Could you check a few things on this model? Use its own coordinates, in mm. A direction names the side the tool comes from. Coordinates: 2 decimals unless noted, no trailing zeros. Write each loop counter-clockwise with the first axis right and the second up, starting at its lowest first coordinate (ties: lowest second). Pieces come first, ordered by that corner, then holes.
```python
from build123d import *

# Parameters (mm, degrees)
F2_R     = 1.5
F3_DEPTH = 4
F5_DEPTH = 1.5


with BuildPart() as f1:
    # F0 (on Right) → F1 (revolve)
    with BuildSketch(Plane.YZ):
        with BuildLine():
            Line((0, 0), (0, 6))
            ThreePointArc((0, 6), (-1.1189941578, 3.0922762594), (-1.4995632221, 0))
            Line((-1.4995632221, 0), (0, 0))
        make_face()
    revolve(axis=Axis((0, 0.9339665994, 0), (0, 1, 0)))

    # F2 (on Front) → F3 (join)
    with BuildSketch(Plane.XZ):
        Circle(F2_R)
    extrude(amount=F3_DEPTH)

    # F4 (on Top) → F5 (join, symmetric)
    with BuildSketch(Plane.XY):
        with BuildLine():
            Line((1.4699705266, -3.8650664501), (0, -3.8650664501))
            Line((0, -3.8650664501), (-1.4699705266, -3.8650664501))
            ThreePointArc((-1.4699705266, -3.8650664501), (-2.105403361, -4.0929103047), (-2.4512772628, -4.6726162242))
            Line((-2.4512772628, -4.6726162242), (-5.0702010152, -18.0265497334))
            ThreePointArc((-5.0702010152, -18.0265497334), (-5.0479765813, -18.5021273815), (-4.8083588564, -18.913529096))
            Line((-4.8083588564, -18.913529096), (-2.5877873591, -21.213825008))
            ThreePointArc((-2.5877873591, -21.213825008), (-2.2591365885, -21.4397656254), (-1.8683227817, -21.5192958713))
            Line((-1.8683227817, -21.5192958713), (0, -21.5192958713))
            Line((0, -21.5192958713), (1.8683227817, -21.5192958713))
            ThreePointArc((1.8683227817, -21.5192958713), (2.2591365885, -21.4397656254), (2.5877873591, -21.213825008))
            Line((2.5877873591, -21.213825008), (4.8083588564, -18.913529096))
            ThreePointArc((4.8083588564, -18.913529096), (5.0479765813, -18.5021273815), (5.0702010152, -18.0265497334))
            Line((5.0702010152, -18.0265497334), (2.4512772628, -4.6726162242))
            ThreePointArc((2.4512772628, -4.6726162242), (2.105403361, -4.0929103047), (1.4699705266, -3.8650664501))
        make_face()
    extrude(amount=F5_DEPTH, both=True)


solid = f1.part
```
1. I want a section at B-B on y = -6.25. Please give me the cut outline in (x, z).
Verdict:
outline: (-2.76, -1.5) - (2.76, -1.5) - (2.76, 1.5) - (-2.76, 1.5) - close
2. I want a section at D-D on z = 3.5. Please give me the cut outline in (x, y), plus the area to 3 significant figures.
Verdict:
outline: (-4.87, 0) arc R12.26 ccw to (4.87, 0) - close
area: 6.62 mm2
3. I want a section at A-A on z = 0. Please give me the cut outline in (x, y).
Verdict:
outline: (-6, 0) arc R12.75 ccw to (-1.5, -1.41) - (-1.5, -3.87) arc R1 ccw to (-2.45, -4.67) - (-5.07, -18.03) arc R1 ccw to (-4.81, -18.91) - (-2.59, -21.21) arc R1 ccw to (-1.87, -21.52) - (1.87, -21.52) arc R1 ccw to (2.59, -21.21) - (4.81, -18.91) arc R1 ccw to (5.07, -18.03) - (2.45, -4.67) arc R1 ccw to (1.5, -3.87) - (1.5, -1.41) arc R12.75 ccw to (6, 0) - close
4. On a 3-axis mill with a long thin cutter (end or side, diameter ignored), from which of +Z, -Z, +X, -X, +Y, -Y can I reach the whole of each face in a straight line? I mean faces 1 (the face through (3.78, -11.44, 0.02)), 2 (the face through (1.2, -3.865, -1.2)), 3 (the face through (-3.742, -11.256, 0.021)). Say none if no direction works.
Verdict:
face 1: +Z, -Z, +X
face 2: -Z, +X
face 3: +Z, -Z, -X
5. I want a section at C-C on z = -1.25. Please give me the cut outline in (x, y).
Verdict:
outline: (-5.87, 0) arc R12.69 ccw to (-0.83, -1.41) - (-0.83, -3.87) - (-1.47, -3.87) arc R1 ccw to (-2.45, -4.67) - (-5.07, -18.03) arc R1 ccw to (-4.81, -18.91) - (-2.59, -21.21) arc R1 ccw to (-1.87, -21.52) - (1.87, -21.52) arc R1 ccw to (2.59, -21.21) - (4.81, -18.91) arc R1 ccw to (5.07, -18.03) - (2.45, -4.67) arc R1 ccw to (1.47, -3.87) - (0.83, -3.87) - (0.83, -1.41) arc R12.69 ccw to (5.87, 0) - close
6. Please list where these lines run through material, in increasing order: line 1 along Z through (x, y) = (4, -18.75); line 2 along Y through (x, z) = (-2, 1.75); line 3 along Y through (x, z) = (0.5, -5.5).
Verdict:
line 1: z = -1.5 to 1.5
line 2: y = -1.22 to 0
line 3: y = -0.24 to 0
7. For pin 1 (6 mm diameter, centred on x = 1.5, y = -19, fed in from +Z); pin 2 (1 mm diameter, centred on y = -12.5, z = -0.5, fed in from -X); pin 3 (1.5 mm diameter, centred on y = -7, z = -2.5, fed in from +X); pin 4 (3 mm diameter, centred on y = -4.5, z = 1, fed in from +X), each with a flat end and sliding along its axis, tell me the tip position at first contact or that it passes through.
Verdict:
pin 1: stops at z = 1.5
pin 2: stops at x = -4.08
pin 3: passes through
pin 4: stops at x = 2.71
